```python
from build123d import *

# Parameters (mm, degrees)
F0_R     = 9.525
F1_DEPTH = 44.45
F3_DEPTH = 25.4
F4_ANGLE = -90


with BuildPart() as f1:
    # F0 (on Top) → F1 (new body)
    with BuildSketch(Plane.XY):
        with BuildLine():
            Line((-12.1103564769, -65.08749924), (-12.1103564769, 23.81250076))
            ThreePointArc((-12.1103564769, 23.81250076), (-44.6307406585, 37.2828849416), (-31.1603564769, 4.76250076))
            ThreePointArc((-31.1603564769, 4.76250076), (-26.6702284164, 2.9026288205), (-24.8103564769, -1.58749924))
            Line((-24.8103564769, -1.58749924), (-24.8103564769, -65.08749924))
            Line((-24.8103564769, -65.08749924), (-12.1103564769, -65.08749924))
        make_face()
        with Locations((-31.1603564769, 23.81250076)):
            Circle(F0_R, mode=Mode.SUBTRACT)
    extrude(amount=F1_DEPTH)

    # F2 (on face) → F3 (cut)
    with BuildSketch(Plane(origin=(-24.8103564769, 0, 0), x_dir=(0, -1, 0), z_dir=(-1, 0, 0))):
        with BuildLine():
            Line((14.28749924, 14.2748), (65.08749924, 14.2748))
            Line((65.08749924, 14.2748), (65.08749924, 30.1498))
            Line((65.08749924, 30.1498), (14.28749924, 30.1498))
            ThreePointArc((14.28749924, 30.1498), (6.34999924, 22.2123), (14.28749924, 14.2748))
        make_face()
        with BuildLine():
            Line((65.08749924, 44.45), (55.56249924, 44.45))
            ThreePointArc((55.56249924, 44.45), (62.2976913308, 41.6601920908), (65.08749924, 34.925))
            Line((65.08749924, 34.925), (65.08749924, 44.45))
        make_face()
        with BuildLine():
            ThreePointArc((65.08749924, 9.525), (62.2976913308, 2.7898079092), (55.56249924, 0))
            Line((55.56249924, 0), (65.08749924, 0))
            Line((65.08749924, 0), (65.08749924, 9.525))
        make_face()
    extrude(amount=-F3_DEPTH, mode=Mode.SUBTRACT)


with BuildPart() as f1_1:
    # F4: moved
    add(f1.part.rotate(Axis((-12.1103564769, 23.81250076, 22.225), (0, 0, -1)), F4_ANGLE))


solid = f1_1.part
```
Source: CAD feature listing. Evaluate the final solid. Frame: model axes, mm. A direction names the side the tool comes from. Round coordinates to 2 decimals unless told otherwise and drop trailing zeros. Loops run counter-clockwise (first coordinate to the right, second up) from the corner with the lowest first, then second, coordinate; pieces in that order, holes last.
(1) Contact query for flat-ended pins moving along their axis: pin 1 Ø5 at (y, z) = (16, 17) entering from -X; pin 2 Ø4 at (x, z) = (-10, 8.5) entering from -Y; pin 3 Ø6 at (x, y) = (12.5, 15.5) entering from -Z; pin 4 Ø5 at (y, z) = (20, 19) entering from -X. Output: stop coordinate, or through.
From the geometry:
pin 1: stops at x = -29.04
pin 2: stops at y = -14.29
pin 3: stops at z = 0
pin 4: stops at x = -26.28
(2) Pull-direction query (X, two-part tool) for faces 4 (the flat face through (51, 17, 14.275)), 5 (the cylindrical face through (-2.81, 2.7, 21.91)), 6 (the cylindrical face through (74.07, 17.37, 2.86)); classes: +X half, -X half, draft (parallel to the pull), parting line (faces both ways), or undercut.
From the geometry:
face 4: draft
face 5: undercut
face 6: +X half
(3) Access query for faces 1 (the flat face through (45, 11.113, 12)), 2 (the cylindrical face through (-26.018, -8.256, 21.914)), 3 (the flat face through (52, 17, 30.15)). Directions: +Z, -Z, +X, -X, +Y, -Y. A direction counts if a zero-diameter tool reaches every point of the face in a straight line with its end or side. Return the directions, or none.
From the geometry:
face 1: +Z, -Z, +X, -Y
face 2: +Z, -Z
face 3: +X, +Y, -Y
(4) Section query A-A (x = 37.5). Output: boundary loops of the cut face in (y, z).
From the geometry:
outline: (11.11, 0) - (23.81, 0) - (23.81, 14.27) - (11.11, 14.27) - close; (11.11, 30.15) - (23.81, 30.15) - (23.81, 44.45) - (11.11, 44.45) - close
(5) Section query D-D (y = -10). Output: boundary loops of the cut face in (x, z).
From the geometry:
outline: (-24.15, 0) - (-0.07, 0) - (-0.07, 44.45) - (-24.15, 44.45) - close
(6) Material intervals for probe 1 along Z at (x, y) = (48.5, 17); probe 2 along Y at (x, z) = (13, 17); probe 3 along Y at (x, z) = (-18, 36), sorted ascending.
From the geometry:
probe 1: z = 0 to 14.27, 30.15 to 44.45
probe 2: y = 11.11 to 23.81
probe 3: y = -13.35 to -2.72, 12.25 to 22.88
(7) Section query B-B (y = 3). Output: boundary loops of the cut face in (x, z), and give its area (3 significant figures).
From the geometry:
outline: (-31.08, 0) - (-21.47, 0) - (-21.47, 44.45) - (-31.08, 44.45) - close; (-2.75, 0) - (6.86, 0) - (6.86, 44.45) - (-2.75, 44.45) - close
area: 854 mm2
